Part model, mm, in its own coordinate system. Face numbers are marked on the shaded views. Round coordinates to 2 decimals unless told otherwise and drop trailing zeros. Loops run counter-clockwise (first coordinate to the right, second up) from the corner with the lowest first, then second, coordinate; pieces in that order, holes last.
(1) Cut at A-A on x = 13.75. List the corners of the cut face in (y, z), then the cut area to 3 significant figures.
(2) Probe probe 1 along Y at (x, z) = (10, 47); probe 2 along X at (y, z) = (14, 76.5); probe 3 along X at (y, z) = (0.9, 123.5). List the from-to ranges inside material, lowest first.
(3) Cut at C-C on z = 123.5. List the corners of the cut face in (x, y).
(4) Cut at D-D on z = 66.5. List the corners of the cut face in (x, y), then the cut area to 3 significant figures.
(5) Mould opens along Y. For the marked faces 1 and 2 say: +Y half, -Y half, draft (parallel to the pull), parting line (faces both ways), or undercut.
(6) Cut at B-B on z = 163.5. List the corners of the cut face in (x, y).
(7) Flat gauge pins, fed straight in: pin 1 (1 mm diameter, centred on x = 19.5, z = 44.5, fed in from +Y); pin 2 (12 mm diameter, centred on x = 2.5, y = 5.5, fed in from -Z); pin 3 (4.5 mm diameter, centred on y = 10, z = 163.5, fed in from -X); pin 4 (1 mm diameter, centred on x = 19.5, z = 46, fed in from -Y). Where does each tip first touch, or does it go through?
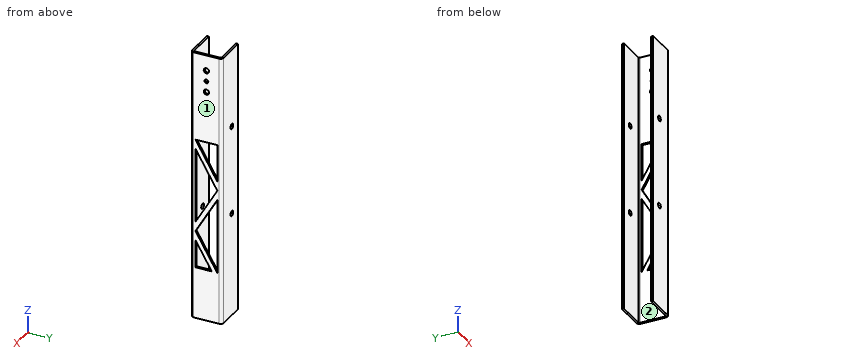
from build123d import *

# Parameters (mm, degrees)
SKETCH1_W                = 20
SKETCH1_H                = 20
BOSS_EXTRUDE1_DEPTH      = 173.5
CONVERT_SOLID1_DEPTH     = 173.5
CUT_EXTRUDE2_DEPTH       = 10
SKETCH15_W               = 56.851586871
SKETCH15_H               = 15.11
BOSS_EXTRUDE2_DEPTH      = 1.29
M3_CLEARANCE_HOLE1_D     = 3.4
M3_CLEARANCE_HOLE1_DEPTH = 3.34
M3_CLEARANCE_HOLE1_TIP   = 1.021463052
SKETCH20_R               = 1.2
CUT_EXTRUDE5_DEPTH       = 5
M3_CLEARANCE_HOLE2_D     = 3.4
SKETCH35_W               = 33.08369384
SKETCH35_H               = 16.22
BOSS_EXTRUDE3_DEPTH      = 1.29


# Read off the part's stored shape, not the designer's step: Convert-Solid1
with BuildPart() as part:
    # Sketch1 → Boss-Extrude1 (new body)
    with BuildSketch(Plane.XY):
        with Locations((10, 10)):
            Rectangle(SKETCH1_W, SKETCH1_H)
    extrude(amount=BOSS_EXTRUDE1_DEPTH)

    # Convert-Solid1 outline → Convert-Solid1 (cut)
    with BuildSketch(Plane.XY):
        with BuildLine():
            Line((20, 0), (20, 1.89))
            ThreePointArc((20, 1.89), (19.446431816, 0.553568184), (18.11, 0))
            Line((18.11, 0), (20, 0))
        make_face()
        with BuildLine():
            ThreePointArc((18.11, 20), (19.446431816, 19.446431816), (20, 18.11))
            Line((20, 18.11), (20, 20))
            Line((20, 20), (18.11, 20))
        make_face()
        with BuildLine():
            Line((0, 18.71), (0, 1.29))
            Line((0, 1.29), (18.11, 1.29))
            ThreePointArc((18.11, 1.29), (18.534264069, 1.465735931), (18.71, 1.89))
            Line((18.71, 1.89), (18.71, 18.11))
            ThreePointArc((18.71, 18.11), (18.534264069, 18.534264069), (18.11, 18.71))
            Line((18.11, 18.71), (0, 18.71))
        make_face()
    extrude(amount=CONVERT_SOLID1_DEPTH, mode=Mode.SUBTRACT)

    # Sketch3 → Cut-Extrude2 (cut)
    with BuildSketch(Plane(origin=(20, 0, 0), x_dir=(0, 0, -1), z_dir=(1, 0, 0))):
        Polygon((-86.75, 17), (-62.796826259, 3), (-110.703173741, 3), align=None)
        Polygon((-80.804760612, 17), (-56.851586871, 3), (-32.898413129, 17), align=None)
        Polygon((-50.906347483, 3), (-26.953173741, 17), (-3, 3), align=None)
        Polygon((-21.007934353, 17), (-3, 6.474836042), (-3, 17), align=None)
        Polygon((-170.5, 17), (-152.492065647, 17), (-170.5, 6.474836042), align=None)
        Polygon((-170.5, 3), (-122.593652517, 3), (-146.546826259, 17), align=None)
        Polygon((-140.601586871, 17), (-92.695239388, 17), (-116.648413129, 3), align=None)
    extrude(amount=-CUT_EXTRUDE2_DEPTH, mode=Mode.SUBTRACT)

    # Sketch15 → Boss-Extrude2 (add)
    with BuildSketch(Plane(origin=(20, 0, 0), x_dir=(0, 0, -1), z_dir=(1, 0, 0))):
        with Locations((-145.074206565, 9.445)):
            Rectangle(SKETCH15_W, SKETCH15_H)
    extrude(amount=-BOSS_EXTRUDE2_DEPTH)

    # M3 Clearance Hole1
    with Locations(Plane.ZY.offset(-18.71)):
        with Locations((163.5, 10), (149.5, 10)):
            Hole(M3_CLEARANCE_HOLE1_D / 2, depth=M3_CLEARANCE_HOLE1_DEPTH)
            with Locations((0, 0, -(M3_CLEARANCE_HOLE1_DEPTH + M3_CLEARANCE_HOLE1_TIP / 2))):  # 118° drill point
                Cone(0, M3_CLEARANCE_HOLE1_D / 2, M3_CLEARANCE_HOLE1_TIP, mode=Mode.SUBTRACT)

    # Sketch20 → Cut-Extrude5 (cut)
    with BuildSketch(Plane.ZY.offset(-18.71)):
        with Locations(Location((156.5, 10, 0), (0, 0, 270))):
            Circle(SKETCH20_R)
    extrude(amount=-CUT_EXTRUDE5_DEPTH, mode=Mode.SUBTRACT)

    # M3 Clearance Hole2 (through all)
    with Locations(Plane(origin=(85.70162808, 20, 101.952320986), x_dir=(0, 0, -1), z_dir=(0, 1, 0))):
        with Locations((-21.547679014, 77.93962808), (35.452320986, 77.93962808)):
            Hole(M3_CLEARANCE_HOLE2_D / 2)

    # Sketch35 → Boss-Extrude3 (add)
    with BuildSketch(Plane(origin=(20, 0, 0), x_dir=(0, 0, -1), z_dir=(1, 0, 0))):
        with Locations((-16.54184692, 10)):
            Rectangle(SKETCH35_W, SKETCH35_H)
    extrude(amount=-BOSS_EXTRUDE3_DEPTH)


solid = part.part
Final values:
1. outline: (0, 0) - (1.29, 0) - (1.29, 173.5) - (0, 173.5) - close; (18.71, 0) - (20, 0) - (20, 173.5) - (18.71, 173.5) - close
1. area: 448 mm2
2. probe 1: y = 0 to 1.29, 18.71 to 20
2. probe 2: x = 18.71 to 20
2. probe 3: x = 0 to 6.06, 9.46 to 19.72
3. outline: (0, 0) - (6.06, 0) - (6.06, 1.29) - (0, 1.29) - close; (0, 18.71) - (6.06, 18.71) - (6.06, 20) - (0, 20) - close; (9.46, 0) - (18.11, 0) arc R1.89 ccw to (20, 1.89) - (20, 18.11) arc R1.89 ccw to (18.11, 20) - (9.46, 20) - (9.46, 18.71) - (18.11, 18.71) arc R0.6 cw to (18.71, 18.11) - (18.71, 1.89) arc R0.6 cw to (18.11, 1.29) - (9.46, 1.29) - close
4. outline: (0, 0) - (6.06, 0) - (6.06, 1.29) - (0, 1.29) - close; (0, 18.71) - (6.06, 18.71) - (6.06, 20) - (0, 20) - close; (9.46, 0) - (18.11, 0) arc R1.89 ccw to (20, 1.89) - (20, 3) - (18.71, 3) - (18.71, 1.89) arc R0.6 cw to (18.11, 1.29) - (9.46, 1.29) - close; (9.46, 18.71) - (18.11, 18.71) arc R0.6 cw to (18.71, 18.11) - (18.71, 17) - (20, 17) - (20, 18.11) arc R1.89 ccw to (18.11, 20) - (9.46, 20) - close; (18.71, 5.16) - (20, 5.16) - (20, 8.64) - (18.71, 8.64) - close
4. area: 50.3 mm2
5. face 1: draft
5. face 2: undercut
6. outline: (0, 0) - (18.11, 0) arc R1.89 ccw to (20, 1.89) - (20, 8.3) - (18.71, 8.3) - (18.71, 1.89) arc R0.6 cw to (18.11, 1.29) - (0, 1.29) - close; (0, 18.71) - (18.11, 18.71) arc R0.6 cw to (18.71, 18.11) - (18.71, 11.7) - (20, 11.7) - (20, 18.11) arc R1.89 ccw to (18.11, 20) - (0, 20) - close
7. pin 1: stops at y = 19.78
7. pin 2: stops at z = 0
7. pin 3: stops at x = 18.71
7. pin 4: stops at y = 0.22
